Build history of the part. All positions in model axes, mm. Coordinates: 2 decimals unless noted, no trailing zeros. Order: outer loops, then holes, each group sorted by start corner. A loop starts at its lowest first (then second) coordinate and runs counter-clockwise, first axis right, second up. Notation, with made-up numbers: (-24, 70.5) - (18, 70.5) arc R9 cw to (18, 85.5) - close; hole circle Ø10 at (83.25, 5). An arc over 180 degrees is marked (long way). One line per item, written item: value.
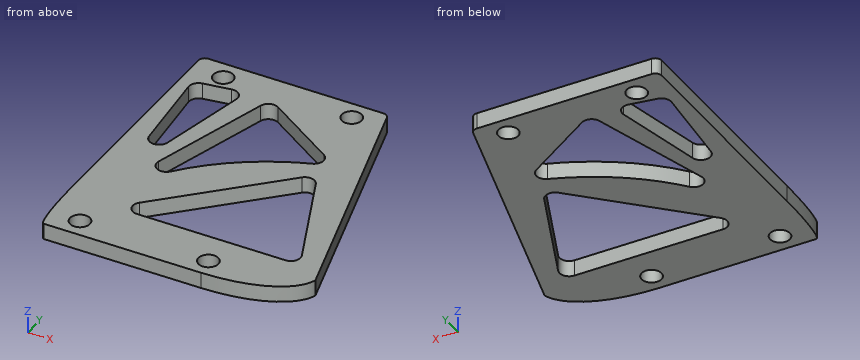
from build123d import *

# Parameters (mm, degrees)
SKETCH_1_R          = 1.55
EXTRUDE_1_DEPTH     = 2.5
CUT_EXTRUDE_1_DEPTH = 50.802108389
FILLET_1_R          = 1.5
FILLET_START        = -1
FILLET_2_DEPTH      = 4
FILLET_3_SIZE       = 10
FILLET_3_SIZE_2     = 1
FILLET_4_R          = 1


with BuildPart() as part:
    # 草图1 → 凸台-拉伸1 (new body)
    with BuildSketch(Plane.XY):
        Polygon((-15, 3), (-15, -3), (25, -3), (25, 3), (14, 43), (-15, 43), (-15, 37), align=None)
        with Locations((-10, 0)):
            Circle(SKETCH_1_R, mode=Mode.SUBTRACT)
        with Locations((10, 0)):
            Circle(SKETCH_1_R, mode=Mode.SUBTRACT)
        with Locations(Location((10, 40, 0), (0, 0, 180))):
            Circle(SKETCH_1_R, mode=Mode.SUBTRACT)
        with Locations(Location((-10, 40, 0), (0, 0, 180))):
            Circle(SKETCH_1_R, mode=Mode.SUBTRACT)
    extrude(amount=EXTRUDE_1_DEPTH)

    # 草图2 → 切除-拉伸1 (cut, through all)
    with BuildSketch(Plane.XY.offset(2.5)):
        with BuildLine():
            Line((-1.665681913, 38.399108294), (13.765828269, 28.537551491))
            add(Edge.make_bspline(
                [(-10.982655732, 6.815263357), (-3.769805813, 23.449653824), (13.765828269, 28.537551491)],
                knots=[0, 0, 0, 1, 1, 1], degree=2))
            Line((-10.982655732, 6.815263357), (-1.665681913, 38.399108294))
        make_face()
        Polygon((-13.170831516, 37.120758338), (-5.409421069, 38.399108294), (-10.982655732, 12.923419887), align=None)
        Polygon((-7.692188848, 5.253320152), (21.344617293, 5.253320152), (12.761410447, 25.524298024), align=None)
    extrude(amount=-CUT_EXTRUDE_1_DEPTH, mode=Mode.SUBTRACT)

    # 圆角1
    fillet_1_edges = [part.edges().sort_by_distance(p)[0] for p in [
        (13.765828269, 28.537551491, 1.25),
        (-10.982655732, 6.815263357, 1.25),
        (-1.665681913, 38.399108294, 1.25),
        (21.344617293, 5.253320152, 1.25),
        (-5.409421069, 38.399108294, 1.25),
        (-10.982655732, 12.923419887, 1.25),
        (-13.170831516, 37.120758338, 1.25),
        (-7.692188848, 5.253320152, 1.25),
        (12.761410447, 25.524298024, 1.25),
    ]]
    fillet(fillet_1_edges, radius=FILLET_1_R)

    # 圆角2: read off the stored shape, not the designer's step
    # 圆角2 outline → 圆角2 (cut)
    with BuildSketch(Plane.XY.offset(FILLET_START)):
        with BuildLine():
            Line((25, -3), (25, 3))
            add(Edge.make_bspline(
                [(25, 3), (23.339885287, -3), (10.543167705, -3)],
                knots=[0, 0, 0, 1, 1, 1], degree=2, weights=[1, 0.795822426, 1]))
            Line((10.543167705, -3), (25, -3))
        make_face()
    extrude(amount=FILLET_2_DEPTH, mode=Mode.SUBTRACT)

    # 圆角3
    # a fillet whose section is not a circle: 10, 1 mm, written as the material it takes off along each edge
    with BuildSketch(Plane(origin=(-15, -3, -25), x_dir=(0, 1, 0), z_dir=(0, 0, 1))) as fillet_3_piece_1:
        with BuildLine():
            Bezier((FILLET_3_SIZE, 0), (0, 0), (0, -FILLET_3_SIZE_2), weights=[1, 0.707106781, 1])
            Line((0, -FILLET_3_SIZE_2), (0, 0))
            Line((0, 0), (FILLET_3_SIZE, 0))
        make_face()
    extrude(amount=52.5, mode=Mode.SUBTRACT)

    # 圆角4
    fillet_4_edges = [part.edges().sort_by_distance(p)[0] for p in [
        (14, 43, 1.25),
        (-15, 43, 1.25),
    ]]
    fillet(fillet_4_edges, radius=FILLET_4_R)


solid = part.part
1. Band-saw the part on C-C, the plane y = 31.5. Give the cut face in (x, z), and give its area (3 significant figures).
Values found:
outline: (-15, 0) - (-12.66, 0) - (-12.66, 2.5) - (-15, 2.5) - close; (-6.92, 0) - (-3.7, 0) - (-3.7, 2.5) - (-6.92, 2.5) - close; (9.13, 0) - (17.16, 0) - (17.16, 2.5) - (9.13, 2.5) - close
area: 34.0 mm2
2. Band-saw the part on A-A, the plane x = -10. Give the cut face in (y, z).
Values found:
outline: (-3, 0) - (-1.55, 0) - (-1.55, 2.5) - (-3, 2.5) - close; (1.55, 0) - (21.31, 0) - (21.31, 2.5) - (1.55, 2.5) - close; (37.64, 0) - (38.45, 0) - (38.45, 2.5) - (37.64, 2.5) - close; (41.55, 0) - (43, 0) - (43, 2.5) - (41.55, 2.5) - close
3. Band-saw the part on B-B, the plane y = 15. Give the cut face in (x, z).
Values found:
outline: (-15, 0) - (2.14, 0) - (2.14, 2.5) - (-15, 2.5) - close; (17.22, 0) - (21.7, 0) - (21.7, 2.5) - (17.22, 2.5) - close
4. Band-saw the part on D-D, the plane z = 1.1. Count the separate pieces of the cut face and the enclosed holes in it, and give its area (3 significant figures).
Values found:
separate pieces: 1
enclosed holes: 7
area: 1,010 mm2
5. Flat gauge pin, fed straight in: P1, Ø10, axis at x = -3.5, y = 27.5, coming from the +Z side. Where does the tip first touch, or does it go through?
Values found:
P1: stops at z = 2.5
6. Probe line 1 along Y through (x, z) = (10, 0.8); line 2 along Y through (x, z) = (-10.5, 1.8); line 3 along Y through (x, z) = (-1.5, 2.05). List the from-to ranges inside material, lowest first.
Values found:
line 1: y = -3 to -1.55, 1.55 to 5.25, 22.79 to 27.27, 30.94 to 38.45, 41.55 to 43
line 2: y = -3 to -1.47, 1.47 to 21.27, 37.56 to 38.53, 41.47 to 43
line 3: y = -3 to 5.25, 11.39 to 20.29, 37.38 to 43
